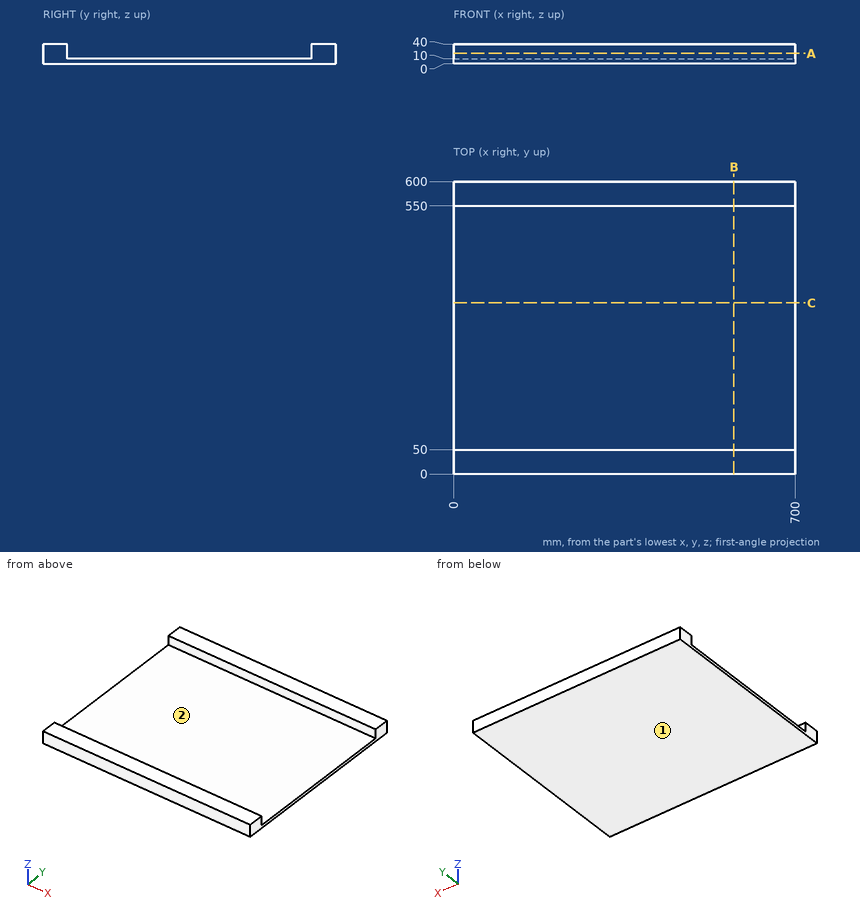
The drawing under review shows one solid part. Ordinate dimensions are in mm from its lowest x, y, z. Coordinates: 2 decimals unless noted, no trailing zeros. Order: outer loops, then holes, each group sorted by start corner. A loop starts at its lowest first (then second) coordinate and runs counter-clockwise, first axis right, second up. Notation, with made-up numbers: (61, 83) -> (96, 83) arc R16 ccw to (96, 110) -> close; hole circle Ø11 at (21.25, 59). An arc over 180 degrees is marked (long way). Answer in a Markdown table with one row per item.
(1) Wall thickness on line 1 along Y through (x, z) = (613, 22); line 2 along Z through (x, y) = (276, 236.5): over which ranges is each line inside the solid? List them lowest first.
Answers:
| item | result |
|---|---|
| line 1 | 0 to 50, 550 to 600 |
| line 2 | 0 to 10 |
(2) Consider section C-C (y = 351). Write out the cut boundary in (x, z), plus the area to 3 significant figures.
Answers:
| item | result |
|---|---|
| outline | (0, 0) -> (700, 0) -> (700, 10) -> (0, 10) -> close |
| area | 7,000 mm² |
(3) The part is to be moulded in two halves that separate along Y. For the marked faces 1 and 2, say which applies: +Y half, -Y half, draft (parallel to the pull), parting line (faces both ways), or undercut.
Answers:
| item | result |
|---|---|
| face 1 | draft |
| face 2 | undercut |
(4) Consider section B-B (x = 574.5). Write out the cut boundary in (y, z).
Answers:
| item | result |
|---|---|
| outline | (0, 0) -> (600, 0) -> (600, 40) -> (550, 40) -> (550, 10) -> (50, 10) -> (50, 40) -> (0, 40) -> close |
(5) Insertion check: pin 1 (5 mm diameter, centred on y = 206, z = 11.5, fed in from +X); pin 2 (2 mm diameter, centred on x = 603.5, y = 244.5, fed in from +Z). Each pin has a flat end and moves straight along its axis. Give the tip position at first contact, or say it passes through.
Answers:
| item | result |
|---|---|
| pin 1 | x = 700 |
| pin 2 | z = 10 |
(6) Consider section A-A (z = 21). Write out the cut boundary in (x, y), plus the area to 3 significant figures.
Answers:
| item | result |
|---|---|
| outline | (0, 0) -> (700, 0) -> (700, 50) -> (0, 50) -> close; (0, 550) -> (700, 550) -> (700, 600) -> (0, 600) -> close |
| area | 70,000 mm² |
